Here's the drawing with two shaded views (mm, measured from the low corner). I have some questions. A direction names the side the tool comes from. Round coordinates to 2 decimals unless told otherwise and drop trailing zeros. Loops run counter-clockwise (first coordinate to the right, second up) from the corner with the lowest first, then second, coordinate; pieces in that order, holes last. Notation, with made-up numbers: (-33.75, 39) -> (21.25, 39) arc R13 ccw to (21.25, 46) -> close; hole circle Ø2 at (57, -32.75). An arc over 180 degrees is marked (long way). Write each question's results on one line, items separated by ' | '. Start each with the question number.
1) For P1, Ø2, axis at y = 2.5, z = 16, coming from the +X side; P2, Ø2, axis at y = 2.5, z = 16.5, coming from the +X side; P3, Ø3, axis at x = 13.5, y = 2.5, coming from the -Z side, each with a flat end and sliding along its axis, tell me the tip position at first contact or that it passes through.
2) Imagine slicing it at C-C, the plane y = 1.2. List the corners of the cut face in (x, z) for me (3 decimals), plus the area to 3 significant figures.
3) If I drill on probe 1 along X at (y, z) = (2.55, 10.5); probe 2 along Y at (x, z) = (5.75, 9); probe 3 along Z at (x, y) = (7.5, 2.25), over which ranges is the centre line in solid material (lowest first)?
4) Which directions (+Z, -Z, +X, -X, +Y, -Y) give clear straight access to the entire face, cutting with the end or side of a thin tool? Please do the marked faces 1 and 2.
5) Imagine slicing it at B-B, the plane z = 4. List the corners of the cut face in (x, y) for me.
6) Imagine slicing it at D-D, the plane x = 19.75. List the corners of the cut face in (y, z) for me.
7) Imagine slicing it at A-A, the plane x = 12.5. List the corners of the cut face in (y, z) for me, plus the area to 3 significant figures.
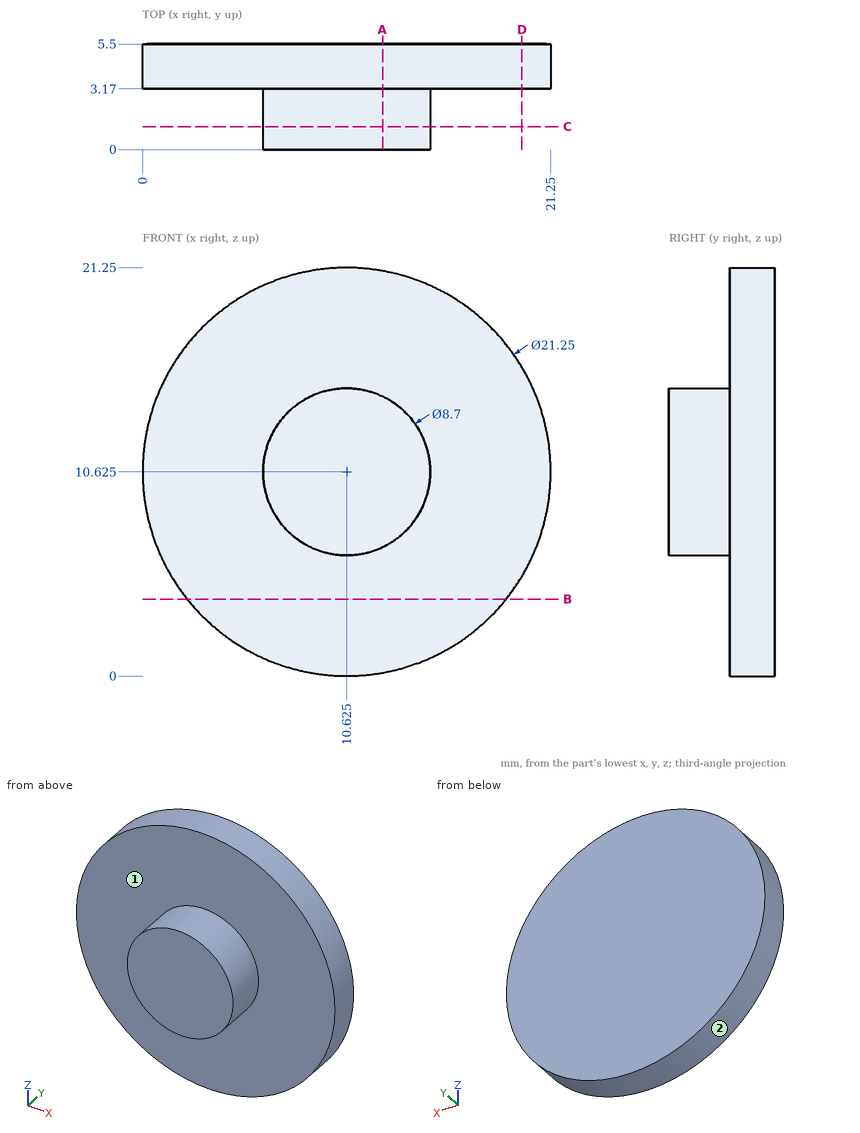
Checked values:
1) P1: x = 20.19 | P2: x = 19.93 | P3: z = 0.11
2) outline: circle Ø8.7 at (10.625, 10.625) | area: 59.4 mm^2
3) probe 1: 6.28 to 14.97 | probe 2: 3.17 to 5.5 | probe 3: 7.6 to 13.65
4) face 1: -Y | face 2: +Y, -Y
5) outline: (2.32, 3.17) -> (18.93, 3.17) -> (18.93, 5.5) -> (2.32, 5.5) -> close
6) outline: (3.17, 5.18) -> (5.5, 5.18) -> (5.5, 16.07) -> (3.17, 16.07) -> close
7) outline: (0, 6.7) -> (3.17, 6.7) -> (3.17, 0.17) -> (5.5, 0.17) -> (5.5, 21.08) -> (3.17, 21.08) -> (3.17, 14.55) -> (0, 14.55) -> close | area: 73.6 mm^2
